```python
from build123d import *

# Parameters (mm, degrees)
SKETCH_W        = 329.5
SKETCH_H        = 198
SKETCH_W_2      = 327.5
SKETCH_H_2      = 196
PAD_DEPTH       = 8
SKETCH001_W     = 329.5
SKETCH001_H     = 198
PAD001_DEPTH    = 2
SKETCH002_W     = 40
SKETCH002_H     = 10
POCKET_DEPTH    = 2.001
CHAMFER_SIZE    = 0.15
CHAMFER001_SIZE = 0.5
CHAMFER002_SIZE = 0.5
SKETCH003_R     = 3
POCKET001_DEPTH = 329.501


with BuildPart() as part:
    # Sketch → Pad (new body)
    with BuildSketch(Plane.XY):
        with Locations((164.75, 99)):
            Rectangle(SKETCH_W, SKETCH_H)
        with Locations((164.75, 99)):
            Rectangle(SKETCH_W_2, SKETCH_H_2, mode=Mode.SUBTRACT)
    extrude(amount=PAD_DEPTH)

    # Sketch001 (on Face9 of Pad) → Pad001 (join)
    with BuildSketch(Plane(origin=(0, 0, 0), x_dir=(1, 0, 0), z_dir=(0, 0, -1))):
        with Locations((164.75, -99)):
            Rectangle(SKETCH001_W, SKETCH001_H)
    extrude(amount=PAD001_DEPTH)

    # Sketch002 (on Face15 of Pad001) → Pocket (cut, through all)
    with BuildSketch(Plane.XY):
        with Locations((207.5, 38)):
            Rectangle(SKETCH002_W, SKETCH002_H)
    extrude(amount=-POCKET_DEPTH, mode=Mode.SUBTRACT)

    # Chamfer
    chamfer_edges = [part.edges().sort_by_distance(p)[0] for p in [
        (207.5, 33, 0),
    ]]
    chamfer(chamfer_edges, length=CHAMFER_SIZE)

    # Chamfer001
    chamfer001_edges = [part.edges().sort_by_distance(p)[0] for p in [
        (207.5, 43, 0),
    ]]
    chamfer(chamfer001_edges, length=CHAMFER001_SIZE)

    # Chamfer002
    chamfer002_edges = [part.edges().sort_by_distance(p)[0] for p in [
        (187.5, 38, -2),
        (227.5, 38, -2),
    ]]
    chamfer(chamfer002_edges, length=CHAMFER002_SIZE)

    # Sketch003 (on Face21 of Chamfer002) → Pocket001 (cut, through all)
    with BuildSketch(Plane(origin=(0, 0, 0), x_dir=(0, -1, 0), z_dir=(-1, 0, 0))):
        with Locations((-193, 4)):
            Circle(SKETCH003_R)
        with Locations((-5, 4)):
            Circle(SKETCH003_R)
    extrude(amount=-POCKET001_DEPTH, mode=Mode.SUBTRACT)


solid = part.part
```
For this review, take the finished solid that the model builds, in its own axes (mm). A direction names the side the tool comes from. Give positions to 0.01 mm unless a question says otherwise; leave off trailing zeros. Write each loop counter-clockwise with the first axis right and the second up, starting at its lowest first coordinate (ties: lowest second). Pieces come first, ordered by that corner, then holes. Notation, with made-up numbers: M -27,-31.5 L 10,-31.5 A16 cw 10,-1.5 Z; hole C 44,41 d5. An arc over 180 degrees is marked long. Answer as a JSON object with one key per item and string values. Group by question number.
Item 1: For probe 1 along Y at (x, z) = (305, 6.75); probe 2 along X at (y, z) = (172, 2.5); probe 3 along Z at (x, y) = (329.1, 5), list the stretches that pass through material, from the lowest coordinate up. Write a range as [from, to].
Item 2: Consider section B-B on y = 69.5. Write out the cut boundary in (x, z).
Item 3: Tool access review of faces 1 (the flat face through (162, 198, 3)), 2 (the flat face through (162, 98, 0)): name each direction out of +Z, -Z, +X, -X, +Y, -Y from which nothing blocks a thin tool from reaching the whole face with its end or side.
Item 4: Consider section A-A on x = 271.5. Write out the cut boundary in (y, z).
Item 5: Consider section C-C on z = 4. Write out the cut boundary in (x, y).
Item 6: Draft analysis for pull direction Z (two halves, no side actions). For faces 3 (the cylindrical face through (0.49, 190.14, 4.9)), 4 (the flat face through (162, 1, 4)), 5 (the flat face through (162, 98, -2)), state which applies: +Z half, -Z half, draft (parallel to the pull), parting line (faces both ways), or undercut.
Item 7: For pin 1 Ø3.5 at (y, z) = (193, 4) entering from +X; pin 2 Ø1 at (x, y) = (113.5, 98) entering from +Z, all flat-tipped, find the tip position at first contact; note any pin that passes through.
Check result:
{
 "1": {"probe 1": "y = [0, 1], [197, 198]", "probe 2": "x = [0, 1], [328.5, 329.5]", "probe 3": "z = [-2, 1], [7, 8]"},
 "2": {"outline": "M 0,-2 L 329.5,-2 L 329.5,8 L 328.5,8 L 328.5,0 L 1,0 L 1,8 L 0,8 Z"},
 "3": {"face 1": "+Z, -Z, +X, -X, +Y", "face 2": "+Z"},
 "4": {"outline": "M 0,-2 L 198,-2 L 198,8 L 197,8 L 197,0 L 1,0 L 1,8 L 0,8 Z"},
 "5": {"outline": "M 0,0 L 329.5,0 L 329.5,2 L 328.5,2 L 328.5,1 L 1,1 L 1,2 L 0,2 Z; M 0,8 L 1,8 L 1,190 L 0,190 Z; M 0,196 L 1,196 L 1,197 L 328.5,197 L 328.5,196 L 329.5,196 L 329.5,198 L 0,198 Z; M 328.5,8 L 329.5,8 L 329.5,190 L 328.5,190 Z"},
 "6": {"face 3": "undercut", "face 4": "draft", "face 5": "-Z half"},
 "7": {"pin 1": "passes through", "pin 2": "stops at z = 0"}
}
